Part print with two shaded views. Sizes in mm from the minimum x, y, z corner. A direction names the side the tool comes from. Give positions to 0.01 mm unless a question says otherwise; leave off trailing zeros. Loops run counter-clockwise (first coordinate to the right, second up) from the corner with the lowest first, then second, coordinate; pieces in that order, holes last. Notation, with made-up numbers: M 20.25,6 L 68.25,6 A8 ccw 68.25,17 Z; hole C -8,71.5 d2. An arc over 180 degrees is marked long. Answer as a JSON object with one key per item and string values. Group by question number.
1. Mould opens along Y. For the marked faces 3, 4 and 5 say: released by +Y, released by -Y, zero draft, split by the parting line, or undercut.
2. 3-axis set-ups, long thin cutter, end or side, ignore diameter. For the marked faces 1 and 2: which of +Z, -Z, +X, -X, +Y, -Y reach the whole face in a straight line?
3. Slice it at D-D (x = 37.5). List the corners of the cut face in (y, z).
4. Slice it at A-A (x = 20.05). List the corners of the cut face in (y, z).
5. Drill centre lines: line 1 along Y through (x, z) = (20.05, 12.25); line 2 along Y through (x, z) = (20.05, 8); line 3 along Z through (x, y) = (24, 6.5). Where is each one in solid material? Low to high. Write a range as [from, to].
6. Drop flat-ended pins along their axis: pin 1 Ø9 at (x, y) = (20.05, 20.05) entering from +Z; pin 2 Ø10 at (x, y) = (19.5, 4) entering from +Z; pin 3 Ø4 at (x, z) = (12, 4) entering from +Y; pin 4 Ø5 at (y, z) = (32.5, 4) entering from -X. Give the stop position or say it passes through.
7. Slice it at C-C (z = 13). List the corners of the cut face in (x, y), then the cut area to 3 significant figures.
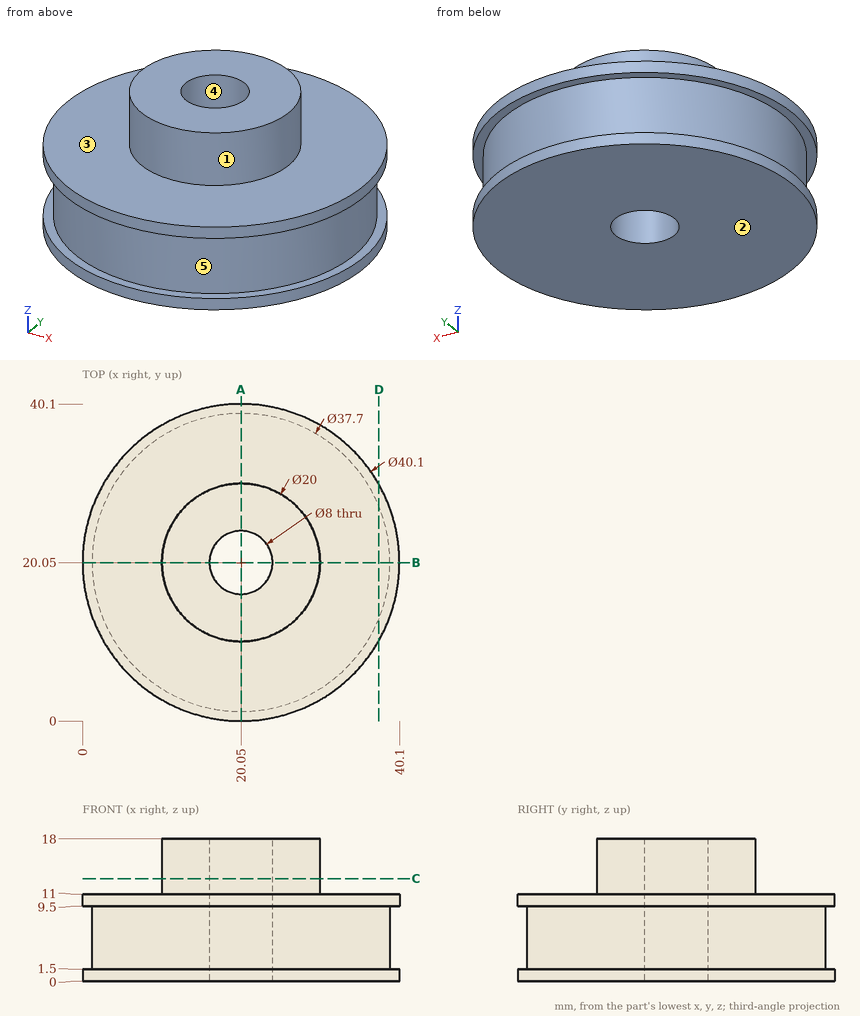
Established:
{
 "1": {"face 3": "zero draft", "face 4": "undercut", "face 5": "split by the parting line"},
 "2": {"face 1": "+Z", "face 2": "-Z, +X, -X, +Y, -Y"},
 "3": {"outline": "M 10.18,0 L 29.92,0 L 29.92,1.5 L 27.18,1.5 L 27.18,9.5 L 29.92,9.5 L 29.92,11 L 10.18,11 L 10.18,9.5 L 12.92,9.5 L 12.92,1.5 L 10.18,1.5 Z"},
 "4": {"outline": "M 0,0 L 16.05,0 L 16.05,18 L 10.05,18 L 10.05,11 L 0,11 L 0,9.5 L 1.2,9.5 L 1.2,1.5 L 0,1.5 Z; M 24.05,0 L 40.1,0 L 40.1,1.5 L 38.9,1.5 L 38.9,9.5 L 40.1,9.5 L 40.1,11 L 30.05,11 L 30.05,18 L 24.05,18 Z"},
 "5": {"line 1": "y = [10.05, 16.05], [24.05, 30.05]", "line 2": "y = [1.2, 16.05], [24.05, 38.9]", "line 3": "z = [0, 11]"},
 "6": {"pin 1": "stops at z = 18", "pin 2": "stops at z = 11", "pin 3": "stops at y = 37.9", "pin 4": "stops at x = 4.04"},
 "7": {"outline": "C 20.05,20.05 d20; hole C 20.05,20.05 d8", "area": "264 mm^2"}
}
